For this review, take the finished solid that the model builds, in its own axes (mm). A direction names the side the tool comes from. Give positions to 0.01 mm unless a question says otherwise; leave off trailing zeros. Order: outer loops, then holes, each group sorted by start corner. A loop starts at its lowest first (then second) coordinate and runs counter-clockwise, first axis right, second up. Notation, with made-up numbers: (63.25, -27.5) - (69.25, -27.5) arc R15 ccw to (69.25, -2.5) - close; hole circle Ø4 at (3.5, 43). An arc over 180 degrees is marked (long way). One line per item, written item: value.
```python
from build123d import *

# Parameters (mm, degrees)
SKETCH1_R           = 33
SKETCH1_R_2         = 28.5
BOSS_EXTRUDE1_DEPTH = 7
SKETCH3_W           = 12
SKETCH3_H           = 9.352768828
BOSS_EXTRUDE2_DEPTH = 7
SKETCH4_R           = 3
CUT_EXTRUDE2_DEPTH  = 3
SKETCH5_R           = 1.6
CUT_EXTRUDE3_DEPTH  = 37
CUT_EXTRUDE4_DEPTH  = 2.5
SKETCH2_W           = 1
SKETCH2_H           = 30
CUT_EXTRUDE1_DEPTH  = 8
SKETCH7_R           = 2.75
BOSS_EXTRUDE3_DEPTH = 7
BOSS_EXTRUDE4_DEPTH = 15
SKETCH9_R           = 1.6
CUT_EXTRUDE5_DEPTH  = 82.669047558
CUT_EXTRUDE6_DEPTH  = 5
FILLET1_R           = 3


with BuildPart() as part:
    # Sketch1 → Boss-Extrude1 (new body)
    with BuildSketch(Plane(origin=(0, 0, 0), x_dir=(1, 0, 0), z_dir=(0, 1, 0))):
        Circle(SKETCH1_R)
        Circle(SKETCH1_R_2, mode=Mode.SUBTRACT)
    extrude(amount=BOSS_EXTRUDE1_DEPTH)

    # Sketch3 → Boss-Extrude2 (add)
    with BuildSketch(Plane(origin=(0, 7, 0), x_dir=(1, 0, 0), z_dir=(0, 1, 0))):
        with Locations((0, -36.323615586)):
            Rectangle(SKETCH3_W, SKETCH3_H)
    extrude(amount=-BOSS_EXTRUDE2_DEPTH)

    # Sketch4 → Cut-Extrude2 (cut)
    with BuildSketch(Plane.ZY.offset(6)):
        with Locations((36.72498074, 3.5)):
            Circle(SKETCH4_R)
    extrude(amount=-CUT_EXTRUDE2_DEPTH, mode=Mode.SUBTRACT)

    # Sketch5 → Cut-Extrude3 (cut, through all)
    with BuildSketch(Plane.ZY.offset(3)):
        with Locations((36.72498074, 3.5)):
            Circle(SKETCH5_R)
    extrude(amount=-CUT_EXTRUDE3_DEPTH, mode=Mode.SUBTRACT)

    # Sketch6 → Cut-Extrude4 (cut)
    with BuildSketch(Plane(origin=(6, 0, 0), x_dir=(0, 0, -1), z_dir=(1, 0, 0))):
        Polygon((-35.137267499, 0.75), (-33.549554259, 3.5), (-35.137267499, 6.25), (-38.31269398, 6.25), (-39.90040722, 3.5), (-38.31269398, 0.75), align=None)
    extrude(amount=-CUT_EXTRUDE4_DEPTH, mode=Mode.SUBTRACT)

    # Sketch2 → Cut-Extrude1 (cut, through all)
    with BuildSketch(Plane(origin=(0, 7, 0), x_dir=(1, 0, 0), z_dir=(0, 1, 0))):
        with Locations((0, -32.66005016)):
            Rectangle(SKETCH2_W, SKETCH2_H)
    extrude(amount=-CUT_EXTRUDE1_DEPTH, mode=Mode.SUBTRACT)

    # Sketch7 → Boss-Extrude3 (add)
    with BuildSketch(Plane(origin=(0, 7, 0), x_dir=(1, 0, 0), z_dir=(0, 1, 0))):
        with Locations((-28.5, 0)):
            Circle(SKETCH7_R)
        with Locations((28.5, 0)):
            Circle(SKETCH7_R)
    extrude(amount=-BOSS_EXTRUDE3_DEPTH)

    # Sketch8 → Boss-Extrude4 (add)
    with BuildSketch(Plane(origin=(0, 0, 0), x_dir=(1, 0, 0), z_dir=(0, 1, 0))):
        Polygon((-26.242146863, -16.184260008), (-16.184260008, -26.242146863), (-19.719793914, -29.777680769), (-29.777680769, -19.719793914), align=None)
    extrude(amount=BOSS_EXTRUDE4_DEPTH)

    # Sketch9 → Cut-Extrude5 (cut, through all)
    with BuildSketch(Plane(origin=(-24.748737342, 0, 24.748737342), x_dir=(0.707106781, 0, 0.707106781), z_dir=(-0.707106781, 0, 0.707106781))):
        with Locations((-3.556, 11)):
            Circle(SKETCH9_R)
        with Locations((3.556, 11)):
            Circle(SKETCH9_R)
    extrude(amount=-CUT_EXTRUDE5_DEPTH, mode=Mode.SUBTRACT)

    # Sketch10 → Cut-Extrude6 (cut)
    with BuildSketch(Plane(origin=(-22.627416998, 0, 22.627416998), x_dir=(0.707106781, 0, 0.707106781), z_dir=(-0.707106781, 0, 0.707106781))):
        Polygon((-0.380573519, 11), (-1.96828676, 13.75), (-5.14371324, 13.75), (-6.731426481, 11), (-5.14371324, 8.25), (-1.96828676, 8.25), align=None)
        Polygon((0.380573519, 11), (1.96828676, 8.25), (5.14371324, 8.25), (6.731426481, 11), (5.14371324, 13.75), (1.96828676, 13.75), align=None)
    extrude(amount=-CUT_EXTRUDE6_DEPTH, mode=Mode.SUBTRACT)

    # Fillet1
    fillet1_edges = [part.edges().sort_by_distance(p)[0] for p in [
        (-17.757230626, 3.5, 27.815117481),
        (-27.815117481, 3.5, 17.757230626),
        (-27.028632172, 7, 16.970745317),
        (-16.970745317, 7, 27.028632172),
    ]]
    fillet(fillet1_edges, radius=FILLET1_R)


solid = part.part
```
(1) Take a section at C-C (x = 1.5). Write out the cut boundary in (y, z), then the cut area to 3 significant figures.
Answers below:
outline: (0, -32.97) - (7, -32.97) - (7, -28.46) - (0, -28.46) - close; (0, 28.46) - (7, 28.46) - (7, 41) - (0, 41) - close; hole circle Ø3.2 at (3.5, 36.72)
area: 111 mm^2
(2) For P1, Ø6, axis at y = 4, z = 38, coming from the +X side; P2, Ø12, axis at x = 6, z = -20, coming from the +Y side; P3, Ø2, axis at y = 4, z = 38, coming from the -X side; P4, Ø3, axis at y = 4, z = 16.5, coming from the +X side, all flat-tipped, find the tip position at first contact; note any pin that passes through.
Answers below:
P1: stops at x = 6
P2: passes through
P3: stops at x = -3
P4: stops at x = 29.39
(3) Draft analysis for pull direction X (two halves, no side actions). For faces 1 (the face through (-3, 4, 41)), 2 (the face through (-17.724, 12.356, 26.137)), 3 (the face through (-26.137, 9.644, 17.724)), state which applies: pulls with the +X half, pulls with the -X half, needs draft (parallel to the pull), parting line crosses it, or undercut.
Answers below:
face 1: needs draft
face 2: undercut
face 3: pulls with the +X half
(4) Machinability: for faces 4 (the face through (-24, 8.25, 19)), 5 (the face through (-0.5, 4, 35)), 6 (the face through (-1.768, 3.57, 35.127)), 7 (the face through (-19.554, 3.451, 20.734)), which of the approach directions +Z, -Z, +X, -X, +Y, -Y give a long, thin tool a straight path to every point of the face, cutting with its end or side? Answer none if there is none.
Answers below:
face 4: none
face 5: +Z, +Y, -Y
face 6: +X, -X
face 7: +Y, -Y
(5) Take a section at B-B (x = 9.5). Write out the cut boundary in (y, z), then the cut area to 3 significant figures.
Answers below:
outline: (0, -31.6) - (7, -31.6) - (7, -26.87) - (0, -26.87) - close; (0, 26.87) - (7, 26.87) - (7, 31.6) - (0, 31.6) - close
area: 66.3 mm^2
(6) Wall thickness on line 1 (Y direction, x = 16.5, z = -26); line 2 (X direction, y = 3.5, z = -20.5); line 3 (X direction, y = 4, z = -1): over which ranges is each line inside the solid? List them lowest first. Write a range as from..to.
Answers below:
line 1: y = 0..7
line 2: x = -25.86..-19.8, 19.8..25.86
line 3: x = -32.98..-25.94, 25.94..32.98
(7) Take a section at A-A (z = 0). Write out the cut boundary in (x, y), then the cut area to 4 significant figures.
Answers below:
outline: (-33, 0) - (-25.75, 0) - (-25.75, 7) - (-33, 7) - close; (25.75, 0) - (33, 0) - (33, 7) - (25.75, 7) - close
area: 101.5 mm^2
